Could you check a few things on this model? Use its own coordinates, in mm. Round coordinates to 2 decimals unless told otherwise and drop trailing zeros. Order: outer loops, then holes, each group sorted by start corner. A loop starts at its lowest first (then second) coordinate and runs counter-clockwise, first axis right, second up. Notation, with made-up numbers: (-7.5, 32.5) - (2.5, 32.5) arc R9 cw to (2.5, 39.5) - close; hole circle Ø10 at (-5.5, 51). An arc over 180 degrees is marked (long way). Use one line per item in the form item = value.
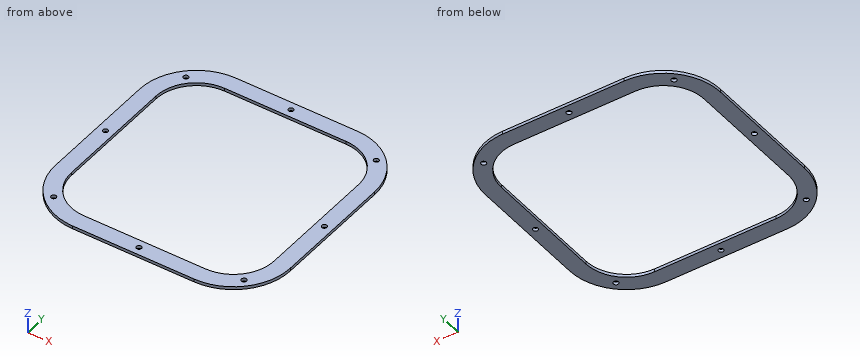
from build123d import *

# Parameters (mm, degrees)
CONVERT_SOLID1_START     = -1.5
CONVERT_SOLID1_OUTLINE_R = 1.25
CONVERT_SOLID1_DEPTH     = 1.5


# Read off the part's stored shape, not the designer's step: Convert-Solid1
with BuildPart() as part:
    # Convert-Solid1 outline → Convert-Solid1 (new body)
    with BuildSketch(Plane.XY.offset(CONVERT_SOLID1_START)):
        with BuildLine():
            Line((116, 28), (116, 88))
            ThreePointArc((116, 88), (107.798989873, 107.798989873), (88, 116))
            Line((88, 116), (28, 116))
            ThreePointArc((28, 116), (8.201010127, 107.798989873), (0, 88))
            Line((0, 88), (0, 28))
            ThreePointArc((0, 28), (8.201010127, 8.201010127), (28, 0))
            Line((28, 0), (88, 0))
            ThreePointArc((88, 0), (107.798989873, 8.201010127), (116, 28))
        make_face()
        with Locations((11.029437252, 11.029437252)):
            Circle(CONVERT_SOLID1_OUTLINE_R, mode=Mode.SUBTRACT)
        with Locations((58, 4)):
            Circle(CONVERT_SOLID1_OUTLINE_R, mode=Mode.SUBTRACT)
        with Locations((104.970562748, 11.029437252)):
            Circle(CONVERT_SOLID1_OUTLINE_R, mode=Mode.SUBTRACT)
        with Locations((4, 58)):
            Circle(CONVERT_SOLID1_OUTLINE_R, mode=Mode.SUBTRACT)
        with Locations((11.029437252, 104.970562748)):
            Circle(CONVERT_SOLID1_OUTLINE_R, mode=Mode.SUBTRACT)
        with BuildLine():
            ThreePointArc((108, 28), (102.142135624, 13.857864376), (88, 8))
            Line((88, 8), (28, 8))
            ThreePointArc((28, 8), (13.857864376, 13.857864376), (8, 28))
            Line((8, 28), (8, 88))
            ThreePointArc((8, 88), (13.857864376, 102.142135624), (28, 108))
            Line((28, 108), (88, 108))
            ThreePointArc((88, 108), (102.142135624, 102.142135624), (108, 88))
            Line((108, 88), (108, 28))
        make_face(mode=Mode.SUBTRACT)
        with Locations((112, 58)):
            Circle(CONVERT_SOLID1_OUTLINE_R, mode=Mode.SUBTRACT)
        with Locations((58, 112)):
            Circle(CONVERT_SOLID1_OUTLINE_R, mode=Mode.SUBTRACT)
        with Locations((104.970562748, 104.970562748)):
            Circle(CONVERT_SOLID1_OUTLINE_R, mode=Mode.SUBTRACT)
    extrude(amount=CONVERT_SOLID1_DEPTH)


solid = part.part
Item 1: Imagine slicing it at A-A on x = 47. Please give me the cut outline in (y, z), plus the area to 3 significant figures.
Found:
outline = (0, -1.5) - (8, -1.5) - (8, 0) - (0, 0) - close; (108, -1.5) - (116, -1.5) - (116, 0) - (108, 0) - close
area = 24.0 mm2
Item 2: Imagine slicing it at C-C on z = -0.75. State how many separate pieces and enclosed holes the cut face has, plus the area to 3 significant figures.
Found:
separate_pieces = 1
enclosed_holes = 9
area = 3,090 mm2
Item 3: Imagine slicing it at B-B on y = 95. Please give me the cut outline in (x, z) (3 decimals), plus the area to 3 significant figures.
Found:
outline = (0.889, -1.5) - (9.265, -1.5) - (9.265, 0) - (0.889, 0) - close; (106.735, -1.5) - (115.111, -1.5) - (115.111, 0) - (106.735, 0) - close
area = 25.1 mm2
Item 4: I need wall thicknesses on L1, parallel to Y at x = 58, z = -0.35; L2, parallel to Y at x = 31, z = -1.3. Which ranges of each line are inside material? Lowest first, please.
Found:
L1 = 0 to 2.75, 5.25 to 8, 108 to 110.75, 113.25 to 116
L2 = 0 to 8, 108 to 116
